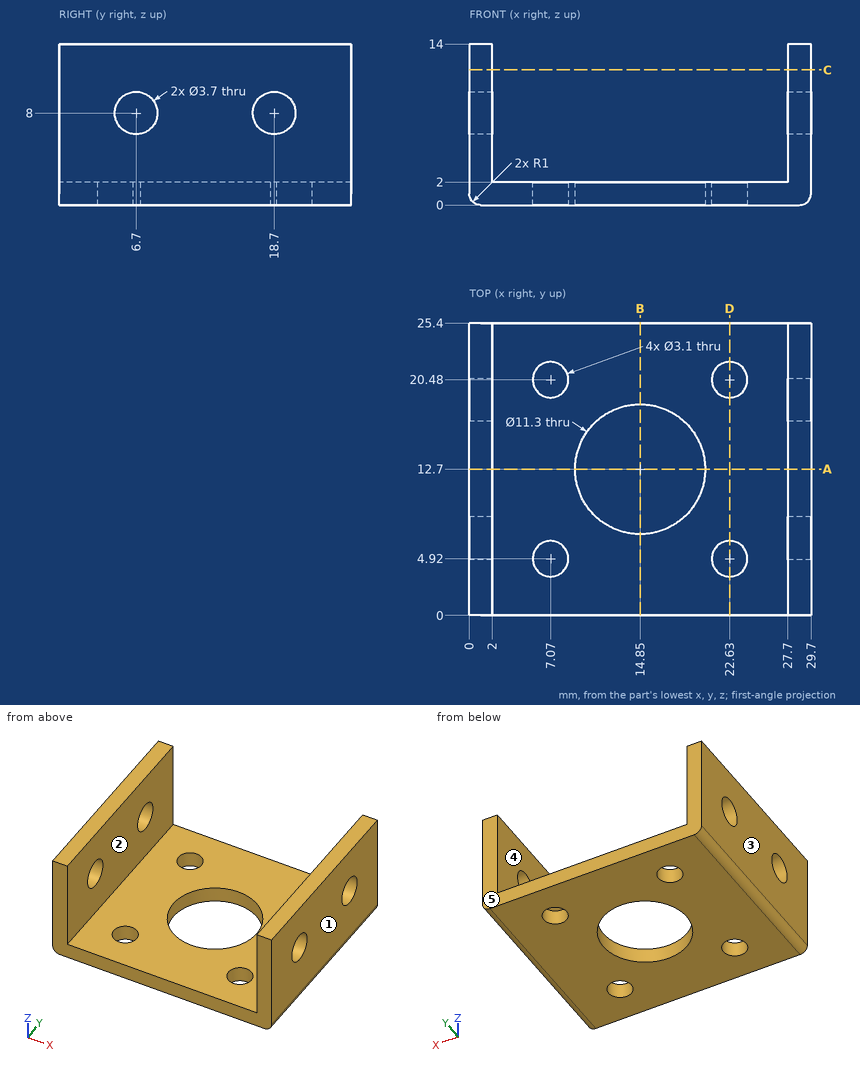
Geometry check sheet. Reference: drawing and pictorial views, mm from the part's lowest x, y, z. A direction names the side the tool comes from. Give positions to 0.01 mm unless a question says otherwise; leave off trailing zeros. Write each loop counter-clockwise with the first axis right and the second up, starting at its lowest first coordinate (ties: lowest second). Pieces come first, ordered by that corner, then holes. Notation, with made-up numbers: (86.5, -12) - (102.5, -12) arc R6 cw to (102.5, -2) - close; hole circle Ø7 at (-40, -32.75). An arc over 180 degrees is marked (long way). Use a Markdown table: item, result.
Q1. Set-up check for the marked faces 1 and 2: record each of +Z, -Z, +X, -X, +Y, -Y from which the full face is reachable in a straight line by a thin tool's end or side.
Computed:
| item | result |
|---|---|
| face 1 | +Z, -Z, +X, +Y, -Y |
| face 2 | +Z, +Y, -Y |
Q2. Section check C-C, the plane z = 11.75. Enter the section's corners in (x, y).
Computed:
| item | result |
|---|---|
| outline | (0, 0) - (2, 0) - (2, 25.4) - (0, 25.4) - close; (27.7, 0) - (29.7, 0) - (29.7, 25.4) - (27.7, 25.4) - close |
Q3. Thickness scan on L1, parallel to Y at x = 7.07, z = 1.65; L2, parallel to Y at x = 0.9, z = 8; L3, parallel to Y at x = 14.85, z = 0.55. Record the ranges inside material, lowest first. Write a range as [from, to].
Computed:
| item | result |
|---|---|
| L1 | y = [0, 3.37], [6.47, 18.93], [22.03, 25.4] |
| L2 | y = [0, 4.85], [8.55, 16.85], [20.55, 25.4] |
| L3 | y = [0, 7.05], [18.35, 25.4] |
Q4. Section check D-D, the plane x = 22.63. Enter the section's corners in (y, z), then the cut area to 3 significant figures.
Computed:
| item | result |
|---|---|
| outline | (0, 0) - (3.37, 0) - (3.37, 2) - (0, 2) - close; (6.47, 0) - (18.93, 0) - (18.93, 2) - (6.47, 2) - close; (22.03, 0) - (25.4, 0) - (25.4, 2) - (22.03, 2) - close |
| area | 38.4 mm² |
Q5. Section check B-B, the plane x = 14.85. Enter the section's corners in (y, z), then the cut area to 3 significant figures.
Computed:
| item | result |
|---|---|
| outline | (0, 0) - (7.05, 0) - (7.05, 2) - (0, 2) - close; (18.35, 0) - (25.4, 0) - (25.4, 2) - (18.35, 2) - close |
| area | 28.2 mm² |
Q6. Section check A-A, the plane y = 12.7. Enter the section's corners in (x, z).
Computed:
| item | result |
|---|---|
| outline | (0, 1) arc R1 ccw to (1, 0) - (9.2, 0) - (9.2, 2) - (2, 2) - (2, 14) - (0, 14) - close; (20.5, 0) - (28.7, 0) arc R1 ccw to (29.7, 1) - (29.7, 14) - (27.7, 14) - (27.7, 2) - (20.5, 2) - close |
Q7. Go/stop test with a flat-tipped pin: P1, Ø5, axis at x = 22, y = 4, coming from the +Z side. Record where the tip stops, or that it passes through.
Computed:
| item | result |
|---|---|
| P1 | stops at z = 2 |
Q8. Draft check along X on the marked faces 3, 4 and 5. Enter one of: pulls with the +X half, pulls with the -X half, needs draft (parallel to the pull), parting line crosses it, or undercut.
Computed:
| item | result |
|---|---|
| face 3 | pulls with the -X half |
| face 4 | undercut |
| face 5 | needs draft |
